Source: three-view drawing plus pictorial views. Frame: mm from the lowest corner of the part. Give positions to 0.01 mm unless a question says otherwise; leave off trailing zeros. Loops run counter-clockwise (first coordinate to the right, second up) from the corner with the lowest first, then second, coordinate; pieces in that order, holes last.
1. Section B-B, the plane y = 5.5. Output: boundary loops of the cut face in (x, z), then the cut area to 3 significant figures.
2. Section A-A, the plane x = 43. Output: boundary loops of the cut face in (y, z), then the cut area to 3 significant figures.
3. First-contact query: P1, Ø3.5, axis at y = 2, z = 5.5, coming from the -X side; P2, Ø1.5, axis at x = 45.5, y = 4.5, coming from the -Z side; P3, Ø6, axis at x = 22, z = 16, coming from the +Y side; P4, Ø1.7, axis at x = 4.5, y = 5.5, coming from the +Z side. Flat tips, straight axial feed; report the tip coordinate or a pass-through.
4. Material intervals for line 1 along X through (y, z) = (0.75, 14.25); line 2 along X through (y, z) = (2.75, 20.75); line 3 along Z through (x, y) = (48.5, 1.25), sorted ascending.
5. Draft query along Z for the marked faces 1, 2 and 3. Return one class per face: +Z half, -Z half, draft (parallel to the pull), parting line (faces both ways), or undercut.
6. Section C-C, the plane y = 1. Output: boundary loops of the cut face in (x, z).
7. Section D-D, the plane x = 4.5. Output: boundary loops of the cut face in (y, z), then the cut area to 3 significant figures.
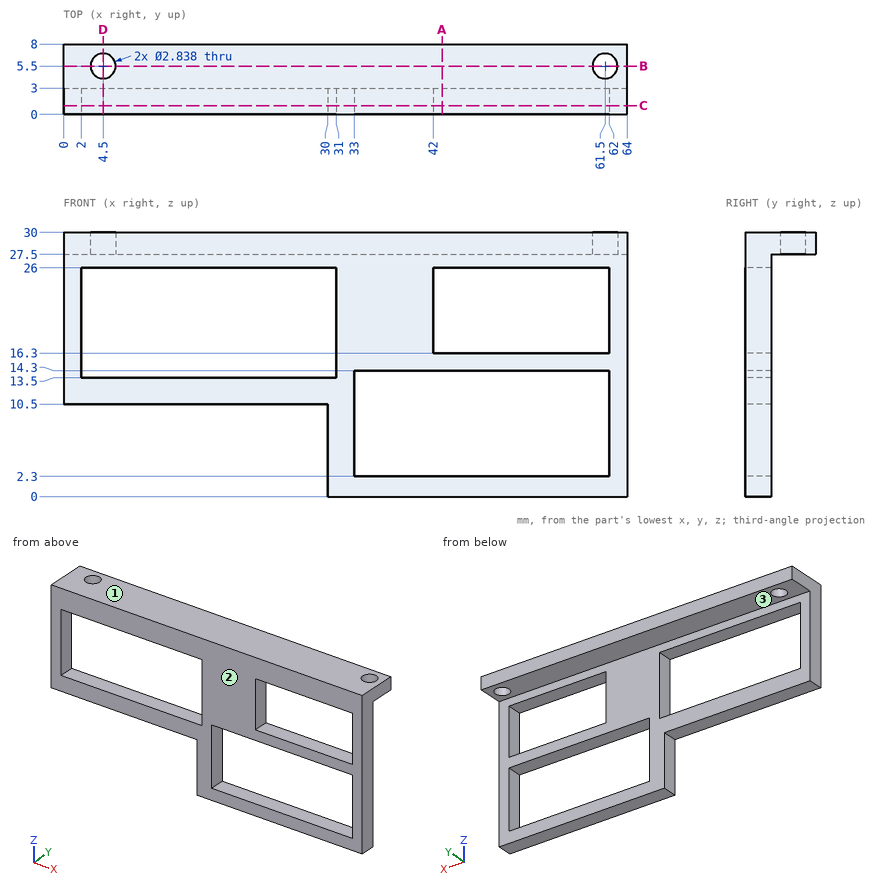
Answers below:
1. outline: (0, 27.5) - (3.08, 27.5) - (3.08, 30) - (0, 30) - close; (5.92, 27.5) - (60.08, 27.5) - (60.08, 30) - (5.92, 30) - close; (62.92, 27.5) - (64, 27.5) - (64, 30) - (62.92, 30) - close
1. area: 146 mm2
2. outline: (0, 0) - (3, 0) - (3, 2.3) - (0, 2.3) - close; (0, 14.3) - (3, 14.3) - (3, 16.3) - (0, 16.3) - close; (0, 26) - (3, 26) - (3, 27.5) - (8, 27.5) - (8, 30) - (0, 30) - close
2. area: 37.4 mm2
3. P1: stops at x = 30
3. P2: stops at z = 27.5
3. P3: stops at y = 3
3. P4: passes through
4. line 1: x = 0 to 2, 31 to 33, 62 to 64
4. line 2: x = 0 to 2, 31 to 42, 62 to 64
4. line 3: z = 0 to 2.3, 14.3 to 16.3, 26 to 30
5. face 1: +Z half
5. face 2: draft
5. face 3: -Z half
6. outline: (0, 10.5) - (30, 10.5) - (30, 0) - (64, 0) - (64, 30) - (0, 30) - close; hole (2, 13.5) - (31, 13.5) - (31, 26) - (2, 26) - close; hole (33, 2.3) - (62, 2.3) - (62, 14.3) - (33, 14.3) - close; hole (42, 16.3) - (62, 16.3) - (62, 26) - (42, 26) - close
7. outline: (0, 10.5) - (3, 10.5) - (3, 13.5) - (0, 13.5) - close; (0, 26) - (3, 26) - (3, 27.5) - (4.08, 27.5) - (4.08, 30) - (0, 30) - close; (6.92, 27.5) - (8, 27.5) - (8, 30) - (6.92, 30) - close
7. area: 26.4 mm2
